The drawing under review shows one solid part. Ordinate dimensions are in mm from its lowest x, y, z. Coordinates: 2 decimals unless noted, no trailing zeros. Order: outer loops, then holes, each group sorted by start corner. A loop starts at its lowest first (then second) coordinate and runs counter-clockwise, first axis right, second up.
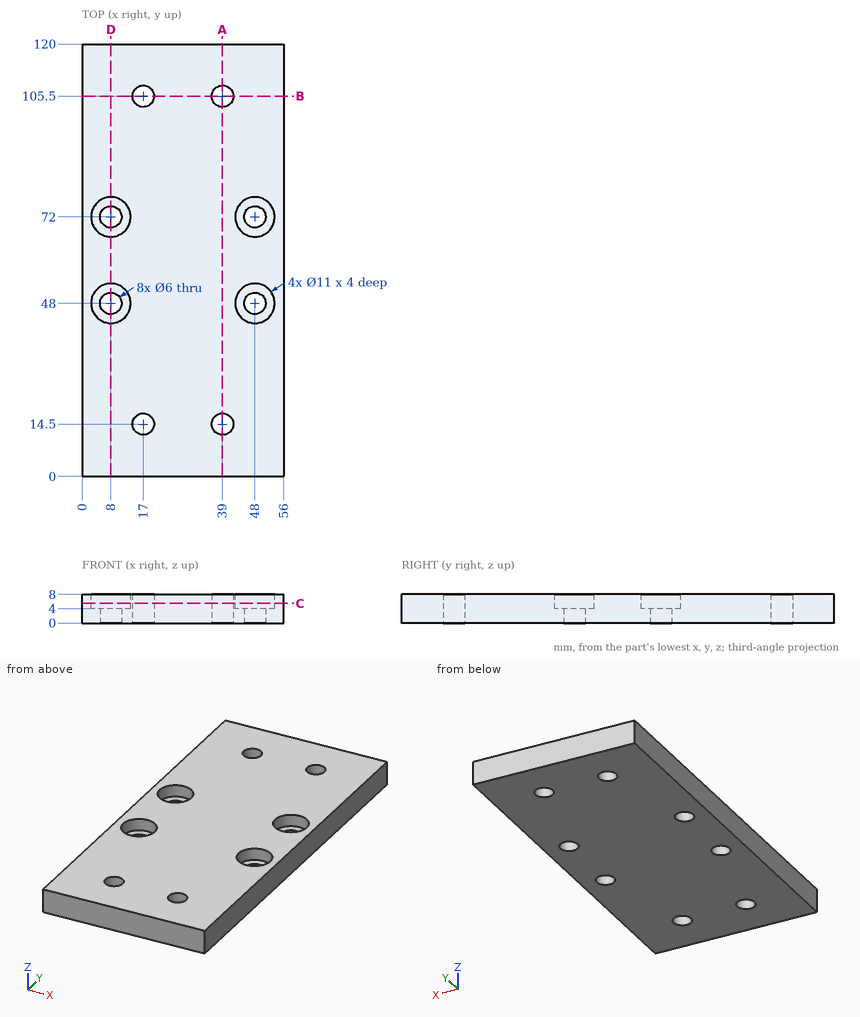
(1) Wall thickness on line 1 (Y direction, x = 48, z = 6.85); line 2 (Y direction, x = 17, z = 2.5); line 3 (X direction, y = 51.5, z = 7.25): over which ranges is each line inside the solid? List them lowest first.
(2) Consider section A-A (x = 39). Give the boundary of the cut face in (y, z), then the cut area to 3 significant figures.
(3) Insertion check: pin 1 Ø3.5 at (x, y) = (48, 48) entering from +Z; pin 2 Ø7 at (x, y) = (8, 48) entering from +Z. Each pin has a flat end and moves straight along its axis. Give the tip position at first contact, or say it passes through.
(4) Consider section B-B (y = 105.5). Give the boundary of the cut face in (x, z).
(5) Consider section C-C (z = 5.5). Give the number of separate pieces and of enclosed holes in the cut face, then the cut area to 3 significant figures.
(6) Consider section D-D (x = 8). Give the boundary of the cut face in (y, z), then the cut area to 3 significant figures.
Findings:
1. line 1: y = 0 to 42.5, 53.5 to 66.5, 77.5 to 120
1. line 2: y = 0 to 11.5, 17.5 to 102.5, 108.5 to 120
1. line 3: x = 0 to 3.76, 12.24 to 43.76, 52.24 to 56
2. outline: (0, 0) - (11.5, 0) - (11.5, 8) - (0, 8) - close; (17.5, 0) - (102.5, 0) - (102.5, 8) - (17.5, 8) - close; (108.5, 0) - (120, 0) - (120, 8) - (108.5, 8) - close
2. area: 864 mm2
3. pin 1: passes through
3. pin 2: stops at z = 4
4. outline: (0, 0) - (14, 0) - (14, 8) - (0, 8) - close; (20, 0) - (36, 0) - (36, 8) - (20, 8) - close; (42, 0) - (56, 0) - (56, 8) - (42, 8) - close
5. separate pieces: 1
5. enclosed holes: 8
5. area: 6,230 mm2
6. outline: (0, 0) - (45, 0) - (45, 4) - (42.5, 4) - (42.5, 8) - (0, 8) - close; (51, 0) - (69, 0) - (69, 4) - (66.5, 4) - (66.5, 8) - (53.5, 8) - (53.5, 4) - (51, 4) - close; (75, 0) - (120, 0) - (120, 8) - (77.5, 8) - (77.5, 4) - (75, 4) - close
6. area: 824 mm2
